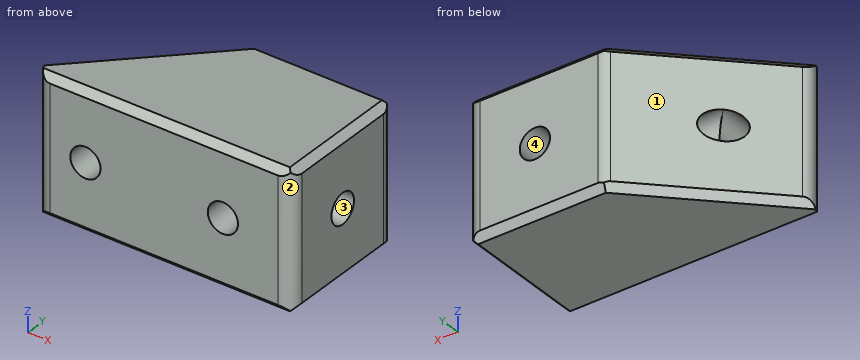
```python
from build123d import *

# Parameters (mm, degrees)
SKETCH1_W                  = 40
SKETCH1_H                  = 20
BOSS_EXTRUDE1_DEPTH        = 20
F_4_4_4_4_DIAMETER_HOLE1_D = 4.4
F_4_4_4_4_DIAMETER_HOLE2_D = 4.4
F_4_4_4_4_DIAMETER_HOLE3_D = 4.4
CUT_EXTRUDE2_DEPTH         = 49.989794856
CHAMFER3_SIZE              = 1
FILLET2_R                  = 2


with BuildPart() as part:
    # Sketch1 → Boss-Extrude1 (new body)
    with BuildSketch(Plane.XY):
        with Locations((20, 10)):
            Rectangle(SKETCH1_W, SKETCH1_H)
    extrude(amount=BOSS_EXTRUDE1_DEPTH)

    # Ø4.4 (4.4) Diameter Hole1 (through all)
    with Locations(Plane.ZY):
        with Locations((10, 10)):
            Hole(F_4_4_4_4_DIAMETER_HOLE1_D / 2)

    # Ø4.4 (4.4) Diameter Hole2 (through all)
    with Locations(Plane(origin=(0, 0, 0), x_dir=(-1, 0, 0), z_dir=(0, -1, 0))):
        with Locations((-30, -10)):
            Hole(F_4_4_4_4_DIAMETER_HOLE2_D / 2)

    # Ø4.4 (4.4) Diameter Hole3 (through all)
    with Locations(Plane(origin=(0, 0, 0), x_dir=(-1, 0, 0), z_dir=(0, -1, 0))):
        with Locations((-10, -10)):
            Hole(F_4_4_4_4_DIAMETER_HOLE3_D / 2)

    # Sketch9 → Cut-Extrude2 (cut, through all)
    with BuildSketch(Plane(origin=(0, 0, 0), x_dir=(-1, 0, 0), z_dir=(0, 0, -1))):
        Polygon((0, 0), (-20, 20), (0, 20), align=None)
    extrude(amount=-CUT_EXTRUDE2_DEPTH, mode=Mode.SUBTRACT)

    # Chamfer3
    chamfer3_edges = [part.edges().sort_by_distance(p)[0] for p in [
        (40, 10, 20),
        (30, 20, 20),
        (10, 10, 20),
        (10, 10, 0),
        (30, 20, 0),
        (40, 10, 0),
        (20, 0, 0),
        (20, 0, 20),
    ]]
    chamfer(chamfer3_edges, length=CHAMFER3_SIZE)

    # Fillet2
    # the kernel refuses this fillet: 2 mm, written as the material it takes off along each edge
    with BuildSketch(Plane(origin=(0, 0, -11.071067812), x_dir=(1, 0, 0), z_dir=(0, 0, 1))) as fillet2_piece_1:
        with BuildLine():
            CenterArc((FILLET2_R * 2.41421356237, FILLET2_R), FILLET2_R, 135, 135)
            Line((FILLET2_R * 1.70710678119, FILLET2_R * 1.70710678119), (0, 0))
            Line((0, 0), (FILLET2_R * 2.41421356237, 0))
        make_face()
    extrude(amount=42.142135624, mode=Mode.SUBTRACT)
    with BuildSketch(Plane(origin=(20, 20, -1.071067812), x_dir=(-0.7071067811865476, -0.7071067811865476, 0), z_dir=(0, 0, 1))) as fillet2_piece_2:
        with BuildLine():
            CenterArc((FILLET2_R * 0.414213562373, FILLET2_R), FILLET2_R, 225, 45)
            Line((-FILLET2_R * 0.292893218813, FILLET2_R * 0.292893218813), (0, 0))
            Line((0, 0), (FILLET2_R * 0.414213562373, 0))
        make_face()
    extrude(amount=22.142135624, mode=Mode.SUBTRACT)
    with BuildSketch(Plane(origin=(40, 20, -4), x_dir=(0, -1, 0), z_dir=(0, 0, 1)), Plane(origin=(40, 0, -4), x_dir=(-1, 0, 0), z_dir=(0, 0, 1))) as fillet2_piece_3:
        with BuildLine():
            CenterArc((FILLET2_R, -FILLET2_R), FILLET2_R, 90, 90)
            Line((0, -FILLET2_R), (0, 0))
            Line((0, 0), (FILLET2_R, 0))
        make_face()
    extrude(amount=28, mode=Mode.SUBTRACT)


solid = part.part
```
Geometry: final body of the model. Coordinates: model frame, mm. Face numbers are marked on the shaded views. Coordinates: 2 decimals unless noted, no trailing zeros. Loops run counter-clockwise (first coordinate to the right, second up) from the corner with the lowest first, then second, coordinate; pieces in that order, holes last. Notation, with made-up numbers: (23.25, 2.5) -> (45.25, 2.5) arc R9 cw to (45.25, 10.5) -> close; hole circle Ø8 at (2.25, 21). An arc over 180 degrees is marked (long way). Use a Markdown table: item, result. Add a question column.
(1) Section query D-D, the plane y = 6.5. Return loops of the section in (x, z), plus the area to 3 significant figures.
(2) Pin query (flat end, axial travel): pin 1 Ø12 at (x, z) = (9.5, 3.5) entering from +Y; pin 2 Ø10 at (y, z) = (16.5, 14) entering from -X; pin 3 Ø2 at (x, z) = (12, 14) entering from +Y. Return the tip coordinate at first contact, or that it passes through.
(3) Line query: line 1 along X through (y, z) = (2.5, 10); line 2 along Z through (x, y) = (36.25, 10); line 3 along X through (y, z) = (2, 11.75). Output: solid intervals per line, ascending.
(4) Mould query, pull axis X, two halves, no side actions, for the marked faces 1, 2, 3 and 4. Classes: pulls with the +X half, pulls with the -X half, needs draft (parallel to the pull), parting line crosses it, or undercut.
(5) Section query B-B, the plane x = 22. Return loops of the section in (y, z).
(6) Section query C-C, the plane x = 29. Return loops of the section in (y, z).
(7) Section query A-A, the plane z = 10. Return loops of the section in (x, y).
Answer:
| question | item | result |
|---|---|---|
| 1 | outline | (6.5, 1) -> (7.91, 0) -> (39, 0) -> (40, 1) -> (40, 19) -> (39, 20) -> (7.91, 20) -> (6.5, 19) -> close; hole circle Ø4.4 at (10, 10); hole circle Ø4.4 at (30, 10) |
| 1 | area | 637 mm^2 |
| 2 | pin 1 | stops at y = 15.5 |
| 2 | pin 2 | stops at x = 11.5 |
| 2 | pin 3 | stops at y = 13 |
| 3 | line 1 | x = 2.89 to 7.8, 12.2 to 27.8, 32.2 to 40 |
| 3 | line 2 | z = 0 to 7.8, 12.2 to 20 |
| 3 | line 3 | x = 2.83 to 8.67, 11.33 to 28.67, 31.33 to 40 |
| 4 | face 1 | pulls with the -X half |
| 4 | face 2 | pulls with the +X half |
| 4 | face 3 | needs draft |
| 4 | face 4 | undercut |
| 5 | outline | (0, 1) -> (1, 0) -> (19, 0) -> (20, 1) -> (20, 19) -> (19, 20) -> (1, 20) -> (0, 19) -> close; hole circle Ø4.4 at (10, 10) |
| 6 | outline | (0, 1) -> (1, 0) -> (19, 0) -> (20, 1) -> (20, 8.04) -> (11, 8.04) arc R2.2 cw to (9, 8.04) -> (0, 8.04) -> close; (0, 11.96) -> (9, 11.96) arc R2.2 cw to (11, 11.96) -> (20, 11.96) -> (20, 19) -> (19, 20) -> (1, 20) -> (0, 19) -> close |
| 7 | outline | (3.41, 3.41) arc R2 ccw to (4.83, 0) -> (7.8, 0) -> (7.8, 7.8) -> close; (12.2, 0) -> (27.8, 0) -> (27.8, 7.8) -> (12.2, 7.8) -> close; (12.2, 12.2) -> (27.8, 12.2) -> (27.8, 20) -> (20.83, 20) arc R2 ccw to (19.41, 19.41) -> close; (32.2, 0) -> (38, 0) arc R2 ccw to (40, 2) -> (40, 7.8) -> (32.2, 7.8) -> close; (32.2, 12.2) -> (40, 12.2) -> (40, 18) arc R2 ccw to (38, 20) -> (32.2, 20) -> close |
